Could you check a few things on this model? Use its own coordinates, in mm. A direction names the side the tool comes from. Round coordinates to 2 decimals unless told otherwise and drop trailing zeros. Loops run counter-clockwise (first coordinate to the right, second up) from the corner with the lowest first, then second, coordinate; pieces in that order, holes last. Notation, with made-up numbers: (-40, -29) - (4, -29) arc R12 cw to (4, -21) - close; hole circle Ø7 at (-32.5, 35). An arc over 180 degrees is marked (long way). Answer as CSV lines item,"result". Start each with the question number.
1) Please list where these lines run through material, in increasing order: line 1 along X through (y, z) = (-20, 61); line 2 along Y through (x, z) = (-33, 28.5); line 3 along Z through (x, y) = (270.5, -3).
2) Suppose I cut it at C-C, the plane y = -10. Write out the boundary of the cut face in (x, z), then the cut area to 3 significant figures.
3) Which directions (+Z, -Z, +X, -X, +Y, -Y) give clear straight access to the entire face, cutting with the end or side of a thin tool? Please do faces 5 (the face through (228.486, -26, 57)), 6 (the face through (-38, -25.4, 57)), 7 (the face through (273, -25, 38.1)), 8 (the face through (-50.914, -13, 57)).
4) Suppose I cut it at D-D, the plane x = 133.5. Write out the boundary of the cut face in (y, z).
5) Suppose I cut it at A-A, the plane z = 42.5. Write out the boundary of the cut face in (x, y).
6) Suppose I cut it at B-B, the plane y = -33. Write out the boundary of the cut face in (x, z), then the cut area to 3 significant figures.
7) I'm going to push flat-ended pins straight in: pin 1 Ø4 at (y, z) = (-34, 66) entering from -X; pin 2 Ø5 at (y, z) = (-38.5, 62) entering from +X; pin 3 Ø7.5 at (x, z) = (-42.5, 56.5) entering from -Y. Where does each tip first touch, or does it pass through?
8) We'd pull the mould along X, two halves only. Please class faces 1 (the face through (-25.514, -13, 57)), 2 (the face through (241, -52.07, 57)), 3 (the face through (72, -25, 38.1)), 4 (the face through (253.886, -26, 57)): pulls with the +X half, pulls with the -X half, needs draft (parallel to the pull), parting line crosses it, or undercut.
```python
from build123d import *

# Parameters (mm, degrees)
F0_W     = 25.4
F0_H     = 38.1
F1_DEPTH = 50.8
F2_DEPTH = 25.4
F3_W     = 25.4
F3_H     = 38.1
F4_DEPTH = 1.27


with BuildPart() as f1:
    # F0 (on Front) → F1 (new body)
    with BuildSketch(Plane.XZ):
        Polygon((-50.914204, 38.1), (-89.014204, 38.1), (-89.014204, 0), (291.985796, 0), (291.985796, 38.1), (253.885796, 38.1), (228.485796, 38.1), (-25.514204, 38.1), align=None)
        with Locations((241.185796, 57.15)):
            Rectangle(F0_W, F0_H)
    extrude(amount=F1_DEPTH)

    # F0 (on Front) → F2 (join)
    with BuildSketch(Plane.XZ):
        with Locations((-38.214204, 57.15)):
            Rectangle(F0_W, F0_H)
    extrude(amount=F2_DEPTH)

    # F3 (on face) → F4 (join)
    with BuildSketch(Plane.XZ.offset(50.8)):
        with Locations((241.185796, 57.15)):
            Rectangle(F3_W, F3_H)
    extrude(amount=F4_DEPTH)


solid = f1.part
```
Filled sheet:
1,line 1,"-50.91 to -25.51, 228.49 to 253.89"
1,line 2,"-50.8 to 0"
1,line 3,"0 to 38.1"
2,outline,"(-89.01, 0) - (291.99, 0) - (291.99, 38.1) - (253.89, 38.1) - (253.89, 76.2) - (228.49, 76.2) - (228.49, 38.1) - (-25.51, 38.1) - (-25.51, 76.2) - (-50.91, 76.2) - (-50.91, 38.1) - (-89.01, 38.1) - close"
2,area,"16,500 mm²"
3,face 5,"+Z, +Y, -Y"
3,face 6,"+Z, -X, -Y"
3,face 7,"+Z, +X, +Y, -Y"
3,face 8,"+Z, -X, +Y, -Y"
4,outline,"(-50.8, 0) - (0, 0) - (0, 38.1) - (-50.8, 38.1) - close"
5,outline,"(-50.91, -25.4) - (-25.51, -25.4) - (-25.51, 0) - (-50.91, 0) - close; (228.49, -52.07) - (253.89, -52.07) - (253.89, 0) - (228.49, 0) - close"
6,outline,"(-89.01, 0) - (291.99, 0) - (291.99, 38.1) - (253.89, 38.1) - (253.89, 76.2) - (228.49, 76.2) - (228.49, 38.1) - (-89.01, 38.1) - close"
6,area,"15,500 mm²"
7,pin 1,"x = 228.49"
7,pin 2,"x = 253.89"
7,pin 3,"y = -25.4"
8,face 1,"undercut"
8,face 2,"needs draft"
8,face 3,"undercut"
8,face 4,"pulls with the +X half"
